```python
from build123d import *

# Parameters (mm, degrees)
SKETCH_1_R          = 5
SKETCH_1_R_2        = 3
EXTRUDE_1_DEPTH     = 5
SKETCH_2_R          = 10
SKETCH_2_R_2        = 3
EXTRUDE_2_DEPTH     = 2
SKETCH_3_R          = 5
EXTRUDE_3_DEPTH     = 3
SKETCH_4_R          = 10
EXTRUDE_4_DEPTH     = 2
SKETCH_5_R          = 3
CUT_EXTRUDE_1_DEPTH = 16.779733838
M3X0_5_1_REACH      = 22.665
M3X0_5_1_BORE_R     = 1.25
SKETCH_7_R          = 1
CUT_EXTRUDE_2_DEPTH = 19.547237056


with BuildPart() as part:
    # ｽｹｯﾁ1 → ﾎﾞｽ - 押し出し1 (new body)
    with BuildSketch(Plane.XY):
        Circle(SKETCH_1_R)
        Circle(SKETCH_1_R_2, mode=Mode.SUBTRACT)
    extrude(amount=EXTRUDE_1_DEPTH)

    # ｽｹｯﾁ2 → ﾎﾞｽ - 押し出し2 (add)
    with BuildSketch(Plane.XY.offset(5)):
        Circle(SKETCH_2_R)
        Circle(SKETCH_2_R_2, mode=Mode.SUBTRACT)
    extrude(amount=EXTRUDE_2_DEPTH)

    # ｽｹｯﾁ3 → ﾎﾞｽ - 押し出し3 (add)
    with BuildSketch(Plane.XY.offset(7)):
        Circle(SKETCH_3_R)
    extrude(amount=EXTRUDE_3_DEPTH)

    # ｽｹｯﾁ4 → ﾎﾞｽ - 押し出し4 (add)
    with BuildSketch(Plane.XY.offset(10)):
        Circle(SKETCH_4_R)
    extrude(amount=EXTRUDE_4_DEPTH)

    # ｽｹｯﾁ5 → ｶｯﾄ - 押し出し1 (cut, through all)
    with BuildSketch(Plane(origin=(0, 0, 7), x_dir=(-1, 0, 0), z_dir=(0, 0, -1))):
        Circle(SKETCH_5_R)
    extrude(amount=-CUT_EXTRUDE_1_DEPTH, mode=Mode.SUBTRACT)

    # M3x0.5 ねじ穴1 bore (on position points) → M3x0.5 ねじ穴1 (cut, up to next)
    with BuildSketch(Plane(origin=(0.251235543, -4.993684081, 2.143915345), x_dir=(-0.998736816219, -0.050247108654, 0), z_dir=(0.050247108654, -0.998736816219, 0)), mode=Mode.PRIVATE) as m3x0_5_1_sk1:
        Circle(M3X0_5_1_BORE_R)
    m3x0_5_1_tool1 = extrude(m3x0_5_1_sk1.sketch, amount=-M3X0_5_1_REACH, mode=Mode.PRIVATE) & part.part
    add(m3x0_5_1_tool1.solids().sort_by_distance((0.251236, -4.993684, 2.143915))[0], mode=Mode.SUBTRACT)

    # ｽｹｯﾁ7 → ｶｯﾄ - 押し出し2 (cut, through all)
    with BuildSketch(Plane.XY.offset(12)):
        with Locations((0.235884413, -6.376305987)):
            Circle(SKETCH_7_R)
    extrude(amount=-CUT_EXTRUDE_2_DEPTH, mode=Mode.SUBTRACT)


solid = part.part
```
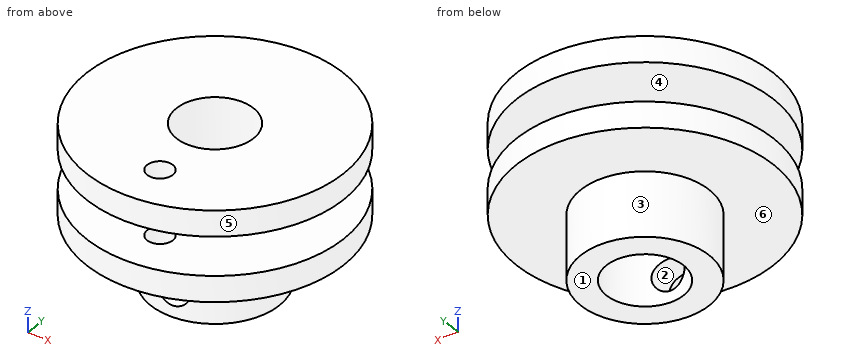
Verification items for the finished model (mm, model axes). Face numbers are marked on the shaded views. A direction names the side the tool comes from. Coordinates: 2 decimals unless noted, no trailing zeros. Order: outer loops, then holes, each group sorted by start corner. A loop starts at its lowest first (then second) coordinate and runs counter-clockwise, first axis right, second up. Notation, with made-up numbers: (82.25, -23.5) -> (89.25, -23.5) arc R24 ccw to (89.25, -4.5) -> close; hole circle Ø4 at (40, 24). An arc over 180 degrees is marked (long way). Put each result on its own line as item: value. Start each with the question number.
1) Go/stop test with flat-tipped pins: pin 1 (1 mm diameter, centred on y = -7.5, z = 6, fed in from -X); pin 2 (4 mm diameter, centred on y = -4, z = 5, fed in from -X); pin 3 (1 mm diameter, centred on x = -6, z = 5.5, fed in from +Y); pin 4 (5 mm diameter, centred on x = 0, y = 0, fed in from -Z). Record where each tip stops, or that it passes through.
2) Cross-section at C-C (y = 0). Enter the section's corners in (x, z), plus the area to 3 significant figures.
3) Cross-section at B-B (x = 6.25). Enter the section's corners in (y, z), plus the area to 4 significant figures.
4) Release check for a two-part mould opening along X. For the marked faces 1, 2 and 3 record: pulls with the +X half, pulls with the -X half, needs draft (parallel to the pull), parting line crosses it, or undercut.
5) Cross-section at D-D (z = 4). Enter the section's corners in (x, y), plus the area to 3 significant figures.
6) Cross-section at A-A (y = 8). Enter the section's corners in (x, z), plus the area to 3 significant figures.
7) Material ranges on L1, parallel to Z at x = 2.25, y = 8.75; L2, parallel to Y at x = 0, z = 4.5; L3, parallel to Y at x = 0, z = 10.4, recorded low to high.
8) Tool access check on the marked faces 4, 5 and 6. Record the directions out of +Z, -Z, +X, -X, +Y, -Y that give a thin tool (end or side, any length) a straight path to the whole face; none if there is none.
Geometry check:
1. pin 1: stops at x = -7.14
1. pin 2: stops at x = -9.8
1. pin 3: stops at y = 8.35
1. pin 4: passes through
2. outline: (-10, 5) -> (-5, 5) -> (-5, 0) -> (-3, 0) -> (-3, 12) -> (-10, 12) -> (-10, 10) -> (-5, 10) -> (-5, 7) -> (-10, 7) -> close; (3, 0) -> (5, 0) -> (5, 5) -> (10, 5) -> (10, 7) -> (5, 7) -> (5, 10) -> (10, 10) -> (10, 12) -> (3, 12) -> close
2. area: 88.0 mm^2
3. outline: (-7.81, 5) -> (7.81, 5) -> (7.81, 7) -> (-7.81, 7) -> close; (-7.81, 10) -> (7.81, 10) -> (7.81, 12) -> (-7.81, 12) -> close
3. area: 62.45 mm^2
4. face 1: needs draft
4. face 2: undercut
4. face 3: parting line crosses it
5. outline: circle Ø10 at (0, 0); hole circle Ø6 at (0, 0)
5. area: 50.3 mm^2
6. outline: (-6, 5) -> (6, 5) -> (6, 7) -> (-6, 7) -> close; (-6, 10) -> (6, 10) -> (6, 12) -> (-6, 12) -> close
6. area: 48.0 mm^2
7. L1: z = 5 to 7, 10 to 12
7. L2: y = -5 to -3, 3 to 5
7. L3: y = -10 to -7.35, -5.4 to -3, 3 to 10
8. face 4: none
8. face 5: +Z, -Z
8. face 6: -Z
